from build123d import *

# Parameters (mm, degrees)
F0_R      = 27.9630212455
F1_DEPTH  = 30
F2_R      = 52.9615929448
F2_R_2    = 27.9630212455
F3_DEPTH  = 35
F4_R      = 34.99999
F5_R      = 9.9870725783
F6_DEPTH  = 110.2
F7_R      = 13.4976595802
F7_R_2    = 9.9870725783
F8_DEPTH  = 10.2
F9_R      = 15.0753999454
F9_R_2    = 13.4976595802
F10_DEPTH = 11.6
F11_R     = 12.993046765
F12_DEPTH = 53
F13_R     = 10.5964364109
F14_DEPTH = 46


# Not quite as in the source:
# - a fillet or chamfer is up to 0.001 mm smaller than in the source, because OpenCascade refuses the exact size


with BuildPart() as f1:
    # F0 (on Front) → F1 (new body)
    with BuildSketch(Plane.XZ):
        with Locations((-0.0335160657, 0.0100570778)):
            Circle(F0_R)
    extrude(amount=F1_DEPTH)

    # F2 (on face) → F3 (join)
    with BuildSketch(Plane.XZ.offset(30)):
        with Locations((-0.0335160657, 0.0100570778)):
            Circle(F2_R)
        with Locations((-0.0335160657, 0.0100570778)):
            Circle(F2_R_2, mode=Mode.SUBTRACT)
        with Locations((-0.0335160657, 0.0100570778)):
            Circle(F2_R_2)
    extrude(amount=F3_DEPTH)

    # F4 (radius 35 in the source; OpenCascade refuses exactly that, so slightly less here)
    f4_edges = [f1.edges().sort_by_distance(p)[0] for p in [
        (-52.995109, -65, 0.010057),
    ]]
    fillet(f4_edges, radius=F4_R)

    # F5 (on face) → F6 (join)
    with BuildSketch(Plane(origin=(0, 0, 0), x_dir=(-1, 0, 0), z_dir=(0, 1, 0))):
        with Locations((0.0335160657, 0.0100570778)):
            Circle(F5_R)
    extrude(amount=F6_DEPTH)

    # F7 (on face) → F8 (join)
    with BuildSketch(Plane(origin=(0, 110.2, 0), x_dir=(-1, 0, 0), z_dir=(0, 1, 0))):
        with Locations((0.0335160657, 0.0100570778)):
            Circle(F7_R)
        with Locations((0.0335160657, 0.0100570778)):
            Circle(F7_R_2, mode=Mode.SUBTRACT)
        with Locations((0.0335160657, 0.0100570778)):
            Circle(F7_R_2)
    extrude(amount=F8_DEPTH)

    # F9 (on face) → F10 (join)
    with BuildSketch(Plane(origin=(0, 120.4, 0), x_dir=(-1, 0, 0), z_dir=(0, 1, 0))):
        with Locations((0.0335160657, 0.0100570778)):
            Circle(F9_R)
        with Locations((0.0335160657, 0.0100570778)):
            Circle(F9_R_2, mode=Mode.SUBTRACT)
        with Locations((0.0335160657, 0.0100570778)):
            Circle(F9_R_2)
    extrude(amount=F10_DEPTH)

    # F11 (on face) → F12 (join)
    with BuildSketch(Plane(origin=(0, 132, 0), x_dir=(-1, 0, 0), z_dir=(0, 1, 0))):
        with Locations((0.0335160657, 0.0100570778)):
            Circle(F11_R)
    extrude(amount=F12_DEPTH)

    # F13 (on face) → F14 (join)
    with BuildSketch(Plane(origin=(0, 185, 0), x_dir=(-1, 0, 0), z_dir=(0, 1, 0))):
        with Locations((0.0335160657, 0.0100570778)):
            Circle(F13_R)
    extrude(amount=F14_DEPTH)


solid = f1.part
Could you check a few things on this model? Use its own coordinates, in mm. A direction names the side the tool comes from. Coordinates: 2 decimals unless noted, no trailing zeros. Loops run counter-clockwise (first coordinate to the right, second up) from the corner with the lowest first, then second, coordinate; pieces in that order, holes last. Notation, with made-up numbers: (-5, -40) -> (-1, -40) arc R19 ccw to (-1, -35) -> close; hole circle Ø8 at (-35, 31.25). An arc over 180 degrees is marked (long way). Answer in a Markdown table with one row per item.
(1) If I drill on probe 1 along Z at (x, y) = (0, 155); probe 2 along X at (y, z) = (-30.5, 5); probe 3 along Y at (x, z) = (-13.5, 45.5), over which ranges is the centre line in solid material (lowest first)?
Results found:
| item | result |
|---|---|
| probe 1 | z = -12.98 to 13 |
| probe 2 | x = -52.76 to 52.69 |
| probe 3 | y = -48.87 to -30 |
(2) Will these pins go through, and if not, where does the flat tip stop? pin 1 Ø5 at (x, y) = (-9, 138.5) entering from -Z; pin 2 Ø12 at (x, z) = (31, 31.5) entering from -Y; pin 3 Ø6 at (y, z) = (27.5, -4.5) entering from -X; pin 4 Ø10 at (x, z) = (10, 9) entering from +Y.
Results found:
| item | result |
|---|---|
| pin 1 | stops at z = -11.26 |
| pin 2 | stops at y = -58.55 |
| pin 3 | stops at x = -9.91 |
| pin 4 | stops at y = 231 |
(3) Imagine slicing it at A-A (y = 102). List the corners of the cut face in (x, z) for me, plus the area to 3 significant figures.
Results found:
| item | result |
|---|---|
| outline | circle Ø19.97 at (-0.03, 0.01) |
| area | 313 mm^2 |
(4) Imagine slicing it at B-B (y = 201.5). List the corners of the cut face in (x, z) for me, plus the area to 3 significant figures.
Results found:
| item | result |
|---|---|
| outline | circle Ø21.19 at (-0.03, 0.01) |
| area | 353 mm^2 |
(5) For faces 5 (the face through (10.68, 115.23, -8.2)), 6 (the face through (12.32, 132, 4.55)), 7 (the face through (0, 231, 0)), which set-ups out of +Z, -Z, +X, -X, +Y, -Y let a thin tool reach every point of the face, with its end or its side?
Results found:
| item | result |
|---|---|
| face 5 | none |
| face 6 | +Y |
| face 7 | +Z, -Z, +X, -X, +Y |
(6) Thinking about a two-plate mould opening in Y: for faces 1 (the face through (-6.095, -14.79, -27.288)), 2 (the face through (12, 0, 0)), 3 (the face through (23, -30, -23)), 4 (the face through (0, -65, 0)), which applies, released by +Y, released by -Y, zero draft, split by the parting line, or undercut?
Results found:
| item | result |
|---|---|
| face 1 | zero draft |
| face 2 | undercut |
| face 3 | released by +Y |
| face 4 | released by -Y |
